The listing builds one solid part. Answer for the finished solid, in the listing's coordinates (mm). Face numbers are marked on the shaded views. A direction names the side the tool comes from. Give positions to 0.01 mm unless a question says otherwise; leave off trailing zeros. Write each loop counter-clockwise with the first axis right and the second up, starting at its lowest first coordinate (ties: lowest second). Pieces come first, ordered by that corner, then holes. Notation, with made-up numbers: M -4.75,-16 L 21.25,-16 A28 ccw 21.25,6 Z; hole C -24,21 d2. An arc over 180 degrees is marked long. Answer as a JSON object with one key per item and string values.
Autodesk Inventor part; units mm, degrees
ref_plane "YZ Plane" through (0, 0, 0) normal (1, 0, 0) x (0, 1, 0)
ref_plane "XZ Plane" through (0, 0, 0) normal (0, 1, 0) x (-1, 0, 0)
ref_plane "XY Plane" through (0, 0, 0) normal (0, 0, 1) x (1, 0, 0)
sketch "Sketch1" plane through (0, 0, 0) normal (0, 0, 1) x (1, 0, 0)
  circle A0 centre (0, 0) radius 6.604
  circle A1 centre (0, 0) radius 16.51
  dimension "d0" = 13.208
  dimension "d1" = 33.02
extrude "Extrusion1" add sketch "Sketch1" along normal blind 6.35
sketch "Sketch2" plane through (0, 0, 6.35) normal (0, 0, 1) x (1, 0, 0)
  circle A0 centre (0, 0) radius 6.604
  circle A1 centre (0, 0) radius 12.7
  dimension "d4" = 25.4
extrude "Extrusion2" add sketch "Sketch2" along normal blind 15.24
sketch "Sketch3" plane through (0, 0, 21.59) normal (0, 0, 1) x (1, 0, 0)
  circle A0 centre (0, 0) radius 12.7
  circle A1 centre (0, 0) radius 16.51
  circle A2 centre (0, 0) radius 6.604
  dimension "d7" = 25.4
  dimension "d8" = 33.02
  dimension "d9" = 13.208
extrude "Extrusion3" add sketch "Sketch3" along normal blind 6.35 contours A0 | A1
sketch "Sketch4" plane through (0, 0, 27.94) normal (0, 0, 1) x (1, 0, 0)
  circle A0 centre (0, 0) radius 6.604
  line L0 (1.3879, 6.604) -> (-1.3553, 6.604)
  line L1 (-1.3553, 6.604) -> (-1.3553, 5.334)
  line L2 (-1.3553, 5.334) -> (1.3879, 5.334)
  line L3 (1.3879, 5.334) -> (1.3879, 6.604)
  point P0 (-2.9121, 5.9273)
  point P1 (-1.3626, 6.604)
  dimension "d12" = 2.7432
  dimension "d13" = 1.27
extrude "Extrusion4" add sketch "Sketch4" against normal blind 27.94 contours L3 L2 L1 A0 | A0 L0 L3 | L1 L0 A0 picked at (0.0109, 5.7573)
sketch "Sketch5" plane through (0, 0, 21.59) normal (0, 0, -1) x (-1, 0, 0)
  arc A0 (-1.3879, 6.4565) -> (1.3553, 6.4634) centre (0, 0) ccw
  circle A1 centre (0, 0) radius 12.7
  circle A2 centre (0, 0) radius 16.1987
  circle A3 centre (0, 0) radius 16.51
  dimension "d16" = 33.02
extrude "Extrusion5" cut sketch "Sketch5" against normal blind 3.175 contours A2 | A3
sketch "Sketch6" plane through (0, 0, 6.35) normal (0, 0, 1) x (1, 0, 0)
  circle A0 centre (0, 0) radius 12.7
  circle A1 centre (0, 0) radius 16.51
  dimension "d19" = 25.4
  dimension "d20" = 33.02
extrude "Extrusion6" cut sketch "Sketch6" against normal blind 3.175
sketch "Sketch7" plane through (0, 0, 3.175) normal (0, 0, 1) x (1, 0, 0)
  circle A0 centre (0, 0) radius 8.89
  circle A1 centre (0, 0) radius 12.7
  dimension "d23" = 17.78
  dimension "d24" = 25.4
extrude "Extrusion7" cut sketch "Sketch7" along normal blind 21.59
chamfer "Chamfer1" distance 3.175 angle 45 4 edges at (-8.89, 0, 3.175) (-16.51, 0, 3.175) (-8.89, 0, 24.765) (-16.51, 0, 24.765)
sketch "Sketch8" plane through (0, 0, 27.94) normal (0, 0, 1) x (1, 0, 0)
  circle A0 centre (0, 0) radius 6.8262
  line L0 (-1.3553, 5.334) -> (-1.3553, 6.4634)
  line L1 (-1.3553, 6.6903) -> (-1.3553, 5.334)
  line L2 (1.3879, 6.4565) -> (1.3879, 5.334)
  line L3 (-1.3553, 5.334) -> (1.3879, 5.334)
  line L4 (1.3879, 5.334) -> (1.3879, 6.6837)
  dimension "d30" = 13.6525
extrude "Extrusion8" cut sketch "Sketch8" against normal blind 50.8 contours A0 L1 L0 L3 L2 L4 picked at (-0.1975, 1.2902)
properties part number "spool"
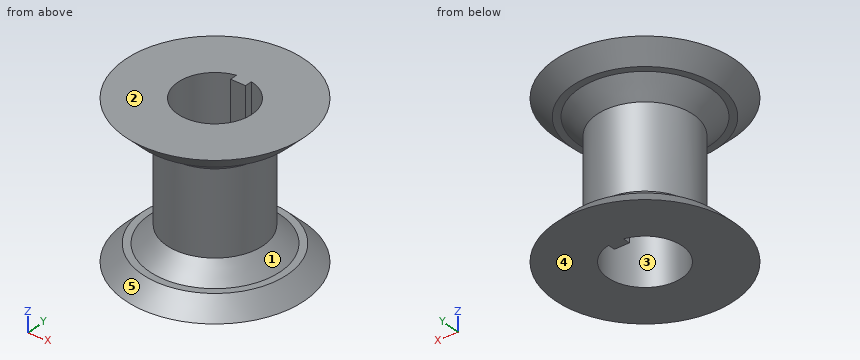
1. For the marked faces 4 and 5, determine the directions among +Z, -Z, +X, -X, +Y, -Y from which every point of the face is accessible in a straight line to the end or side of a thin tool.
Verdict:
{"face 4": "-Z, +X, -X, +Y, -Y", "face 5": "none"}
2. A cutting plane is placed at D-D, the plane z = 23.5. Give the vertices of the cut face in (x, y), plus the area to 3 significant figures.
Verdict:
{"outline": "C 0,0 d21.6; hole M -1.36,5.33 L -1.36,6.69 A6.83 ccw long 1.39,6.68 L 1.39,5.33 Z", "area": "224 mm2"}
3. Consider line 1 along Y through (x, z) = (0, 17.5); line 2 along Z through (x, y) = (0, 13) (3 decimals); line 3 along X through (y, z) = (0, 25.25). Determine where each line is inside the solid, lowest interval first.
Verdict:
{"line 1": "y = -8.89 to -6.83, 5.33 to 8.89", "line 2": "z = 0 to 3.175, 24.765 to 27.94", "line 3": "x = -13.82 to -6.83, 6.83 to 13.82"}
4. A cutting plane is placed at C-C, the plane z = 2.25. Give the vertices of the cut face in (x, y).
Verdict:
{"outline": "C 0,0 d28.52; hole M -1.36,5.33 L -1.36,6.69 A6.83 ccw long 1.39,6.68 L 1.39,5.33 Z"}
5. The mould has two halves that part along Z. Classify the marked faces 1, 2 and 3: released by +Z, released by -Z, zero draft, split by the parting line, or undercut.
Verdict:
{"face 1": "undercut", "face 2": "released by +Z", "face 3": "zero draft"}
6. Flat-ended cylindrical pins translate along their axes: pin 1 (3 mm diameter, centred on y = -10, z = 22.5, fed in from -X); pin 2 (1.5 mm diameter, centred on y = 6.5, z = 12, fed in from -X); pin 3 (2 mm diameter, centred on x = 13, z = 22.5, fed in from -Y); pin 4 (10 mm diameter, centred on x = -13, z = 13, fed in from -Y). Find the tip coordinate at first contact, or state that the pin passes through.
Verdict:
{"pin 1": "stops at x = -6.18", "pin 2": "stops at x = -6.78", "pin 3": "passes through", "pin 4": "stops at y = -3.88"}
